Geometry check sheet. Reference: the model listing, model coordinates, mm. Face numbers are marked on the shaded views. A direction names the side the tool comes from. Coordinates: 2 decimals unless noted, no trailing zeros. Write each loop counter-clockwise with the first axis right and the second up, starting at its lowest first coordinate (ties: lowest second). Pieces come first, ordered by that corner, then holes. Notation, with made-up numbers: (12.5, 72) -> (64.5, 72) arc R20 ccw to (64.5, 89) -> close; hole circle Ø6 at (43.5, 1.25). An arc over 180 degrees is marked (long way). One line per question, with ' | ' between items.
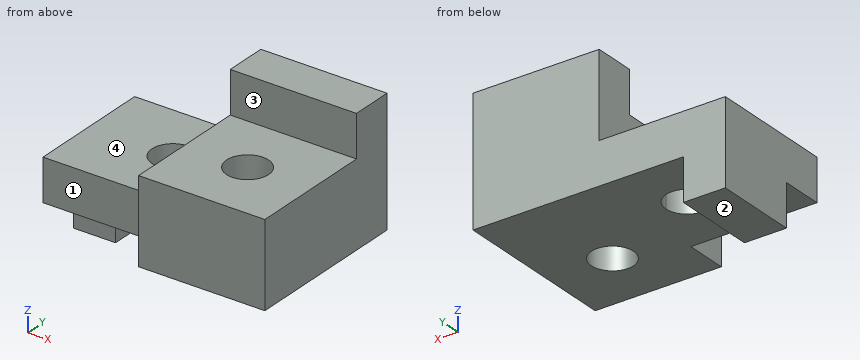
from build123d import *

# Parameters (mm, degrees)
F0_R     = 3.175
F0_W     = 19.05
F0_H     = 6.35
F1_DEPTH = 25.4
F3_DEPTH = 6.35
F4_W     = 6.35
F4_H     = 6.35
F5_DEPTH = 6.35
F6_W     = 19.05
F6_H     = 6.35
F7_DEPTH = 38.1
F8_W     = 19.05
F8_H     = 12.7
F9_DEPTH = 25.4


with BuildPart() as f1:
    # F0 (on Top) → F1 (new body)
    with BuildSketch(Plane.XY):
        Polygon((0, 12.7), (0, 0), (19.05, 0), (19.05, 12.7), (12.7000000394, 12.7), align=None)
        with BuildLine():
            ThreePointArc((15.875, 9.525), (10.4549359558, 7.2799359837), (12.7000000394, 12.7))
            ThreePointArc((12.7000000394, 12.7), (14.9450640442, 11.7700640163), (15.875, 9.525))
        make_face(mode=Mode.SUBTRACT)
        Polygon((19.05, 12.7), (19.05, 0), (19.05, -6.35), (38.1, -6.35), (38.1, 12.7), align=None)
        with Locations((28.575, 3.175)):
            Circle(F0_R, mode=Mode.SUBTRACT)
        Polygon((0, 19.05), (0, 12.7), (12.7000000394, 12.7), (19.05, 12.7), (19.05, 19.05), align=None)
        with Locations((28.575, 15.875)):
            Rectangle(F0_W, F0_H)
    extrude(amount=F1_DEPTH)

    # F2 (on Top) → F3 (cut)
    with BuildSketch(Plane.XY):
        Polygon((38.1, 19.05), (6.35, 19.05), (6.35, 0), (19.05, 0), (19.05, -6.35), (38.1, -6.35), align=None)
    extrude(amount=F3_DEPTH, mode=Mode.SUBTRACT)

    # F4 (on Front) → F5 (cut)
    with BuildSketch(Plane.XZ):
        with Locations((3.175, 3.175)):
            Rectangle(F4_W, F4_H)
    extrude(amount=-F5_DEPTH, mode=Mode.SUBTRACT)

    # F6 (on Right) → F7 (cut)
    with BuildSketch(Plane.YZ):
        with Locations((3.175, 22.225)):
            Rectangle(F6_W, F6_H)
    extrude(amount=F7_DEPTH, mode=Mode.SUBTRACT)

    # F8 (on Front) → F9 (cut)
    with BuildSketch(Plane.XZ):
        with Locations((9.525, 19.05)):
            Rectangle(F8_W, F8_H)
    extrude(amount=-F9_DEPTH, mode=Mode.SUBTRACT)


solid = f1.part
1. Cross-section at B-B on x = 24. Record the boundary of the cut face in (y, z).
Worked answers:
outline: (-6.35, 6.35) -> (19.05, 6.35) -> (19.05, 25.4) -> (12.7, 25.4) -> (12.7, 19.05) -> (-6.35, 19.05) -> close
2. Go/stop test with flat-tipped pins: P1, Ø1.5, axis at x = 15, y = 2, coming from the +Z side; P2, Ø2, axis at x = 28, y = 0, coming from the +Z side; P3, Ø7, axis at x = 2.5, z = 3.5, coming from the -Y side; P4, Ø7, axis at x = 32, z = 22.5, coming from the -Y side. Record where each tip stops, or that it passes through.
Worked answers:
P1: z = 12.7 | P2: z = 19.05 | P3: y = 0 | P4: y = -6.35
3. Cross-section at A-A on y = 13.25. Record the boundary of the cut face in (x, z).
Worked answers:
outline: (0, 0) -> (6.35, 0) -> (6.35, 6.35) -> (38.1, 6.35) -> (38.1, 25.4) -> (19.05, 25.4) -> (19.05, 12.7) -> (0, 12.7) -> close
4. Cross-section at C-C on y = 5.5. Record the boundary of the cut face in (x, z).
Worked answers:
outline: (0, 6.35) -> (26.41, 6.35) -> (26.41, 19.05) -> (19.05, 19.05) -> (19.05, 12.7) -> (0, 12.7) -> close; (30.74, 6.35) -> (38.1, 6.35) -> (38.1, 19.05) -> (30.74, 19.05) -> close
5. Cross-section at D-D on z = 11. Record the boundary of the cut face in (x, y) (3 decimals), and give its area (3 significant figures).
Worked answers:
outline: (0, 0) -> (19.05, 0) -> (19.05, -6.35) -> (38.1, -6.35) -> (38.1, 19.05) -> (0, 19.05) -> close; hole circle Ø6.35 at (12.7, 9.525); hole circle Ø6.35 at (28.575, 3.175) | area: 783 mm²
6. Material ranges on line 1 (X direction, y = 9.5, z = 10); line 2 (Z direction, x = 33.5, y = 12); line 3 (X direction, y = 9, z = 19), recorded low to high. Write a range as from..to.
Worked answers:
line 1: 0..9.53, 15.87..38.1 | line 2: 6.35..19.05 | line 3: 19.05..38.1
7. Tool access check on the marked faces 1, 2, 3 and 4. Record the directions out of +Z, -Z, +X, -X, +Y, -Y that give a thin tool (end or side, any length) a straight path to the whole face; none if there is none.
Worked answers:
face 1: +Z, -Z, -X, -Y | face 2: -Z, +X, -X, +Y, -Y | face 3: +Z, +X, -X, -Y | face 4: +Z, -X, +Y, -Y
